Design review of the part shown in the three views and the two pictorial views. Dimensions are in mm from the part's minimum x, y and z. A direction names the side the tool comes from. Round coordinates to 2 decimals unless told otherwise and drop trailing zeros. Order: outer loops, then holes, each group sorted by start corner. A loop starts at its lowest first (then second) coordinate and runs counter-clockwise, first axis right, second up. Notation, with made-up numbers: M -12.5,82 L 30.5,82 A19 ccw 30.5,116 Z; hole C 39,80.5 d11. An arc over 180 degrees is marked long. Write item = value, one per line. Start each with the question number.
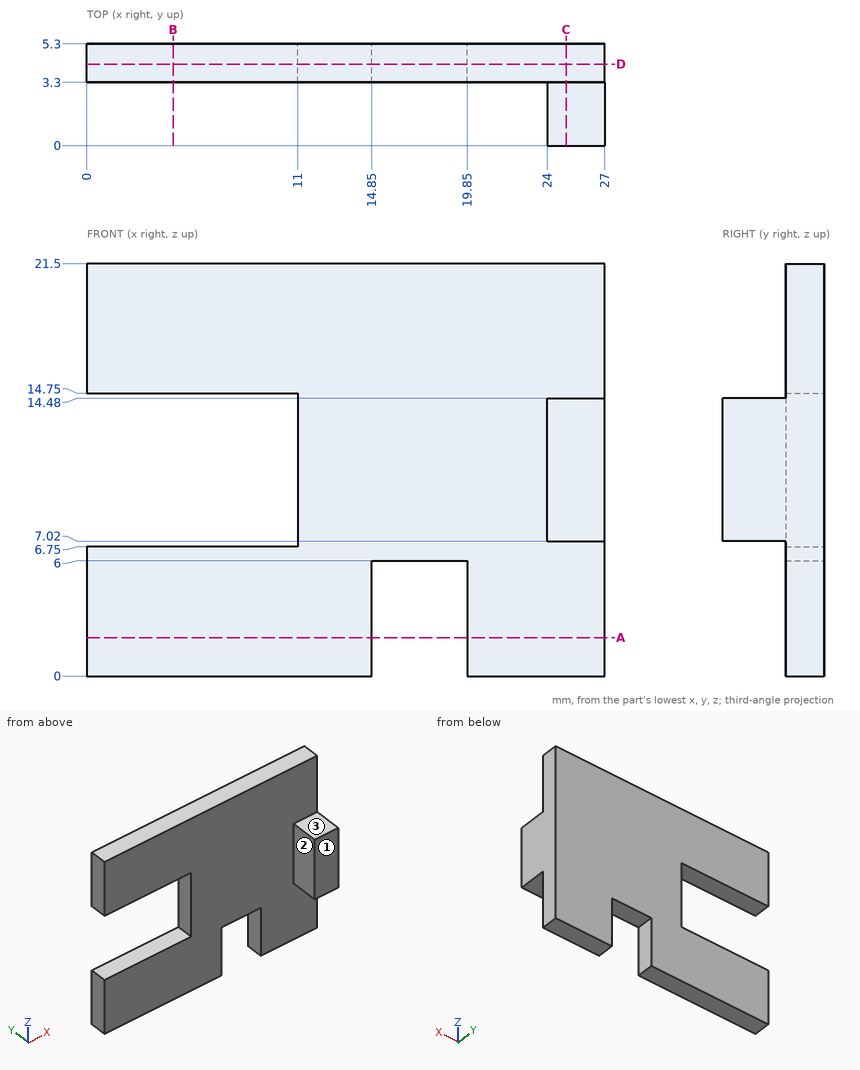
(1) We need section A-A, the plane z = 2. Write out the cut boundary in (x, y).
(2) For the marked faces 1, 2 and 3, list the 3-axis set-ups (+Z, -Z, +X, -X, +Y, -Y) from which the entire face can be reached by the end or side of a thin tool; tool diameter is ignored.
(3) We need section C-C, the plane x = 25. Write out the cut boundary in (y, z).
(4) For line 1 along X through (y, z) = (3.6, 4.75); line 2 along Z through (x, y) = (4, 3.9); line 3 along Y through (x, z) = (23, 18.5), list the stretches that pass through material, from the lowest coordinate up.
(5) We need section B-B, the plane x = 4.5. Write out the cut boundary in (y, z), then the cut area to 3 significant figures.
(6) We need section D-D, the plane y = 4.25. Write out the cut boundary in (x, z).
(7) Insertion check: pin 1 (4 mm diameter, centred on x = 12, z = 17.5, fed in from -Y); pin 2 (2 mm diameter, centred on x = 17, y = 5, fed in from -Z); pin 3 (0.9 mm diameter, centred on x = 25.5, y = 1.5, fed in from -Z). Each pin has a flat end and moves straight along its axis. Give the tip position at first contact, or say it passes through.
Values:
q1.outline = M 0,3.3 L 14.85,3.3 L 14.85,5.3 L 0,5.3 Z; M 19.85,3.3 L 27,3.3 L 27,5.3 L 19.85,5.3 Z
q2.face_1 = +Z, -Z, +X, -X, -Y
q2.face_2 = +Z, -Z, -X, -Y
q2.face_3 = +Z, +X, -X, -Y
q3.outline = M 0,7.02 L 3.3,7.02 L 3.3,0 L 5.3,0 L 5.3,21.5 L 3.3,21.5 L 3.3,14.48 L 0,14.48 Z
q4.line_1 = 0 to 14.85, 19.85 to 27
q4.line_2 = 0 to 6.75, 14.75 to 21.5
q4.line_3 = 3.3 to 5.3
q5.outline = M 3.3,0 L 5.3,0 L 5.3,6.75 L 3.3,6.75 Z; M 3.3,14.75 L 5.3,14.75 L 5.3,21.5 L 3.3,21.5 Z
q5.area = 27.0 mm²
q6.outline = M 0,0 L 14.85,0 L 14.85,6 L 19.85,6 L 19.85,0 L 27,0 L 27,21.5 L 0,21.5 L 0,14.75 L 11,14.75 L 11,6.75 L 0,6.75 Z
q7.pin_1 = 3.3
q7.pin_2 = 6
q7.pin_3 = 7.02
